Design review of the part built by this model. Coordinates are the model's own, in mm. A direction names the side the tool comes from. Coordinates: 2 decimals unless noted, no trailing zeros. Write each loop counter-clockwise with the first axis right and the second up, starting at its lowest first coordinate (ties: lowest second). Pieces come first, ordered by that corner, then holes. Notation, with made-up numbers: (62, -11) - (109, -11) arc R8 ccw to (109, 3) - close; hole circle Ø10 at (19, 1.5). An arc over 180 degrees is marked (long way). Answer as a JSON object with one key per item and string values.
```python
from build123d import *

# Parameters (mm, degrees)
BOSS_EXTRUDE1_DEPTH      = 25
BOSS_EXTRUDE1_DEPTH_BACK = 25
SKETCH2_W                = 1000
SKETCH2_H                = 25.4
CUT_EXTRUDE1_DEPTH       = 762
CUT_EXTRUDE1_DEPTH_BACK  = 762
SKETCH4_W                = 23.68
SKETCH4_H                = 49.713198884
SKETCH5_R                = 2.45
CUT_EXTRUDE2_DEPTH       = 39.05
CUT_EXTRUDE3_DEPTH       = 39.05
CUT_EXTRUDE3_DEPTH_BACK  = 39.05
SKETCH6_R                = 2.4


with BuildPart() as part:
    # Sketch2 → Boss-Extrude1 (new, two sides: drawn at the far end of the back side and taken through both)
    with BuildSketch(Plane(origin=(0, 0, 0), x_dir=(1, 0, 0), z_dir=(0, 1, 0)).offset(-BOSS_EXTRUDE1_DEPTH_BACK)):
        Rectangle(SKETCH2_W, SKETCH2_H)
    extrude(amount=BOSS_EXTRUDE1_DEPTH + BOSS_EXTRUDE1_DEPTH_BACK)

    # Sketch4 → Cut-Extrude1 (cut, two sides: drawn at the far end of the back side and taken through both)
    with BuildSketch(Plane(origin=(0, 0, 0), x_dir=(0, 0, -1), z_dir=(1, 0, 0)).offset(-CUT_EXTRUDE1_DEPTH_BACK)):
        with Locations((0, -0.716599442)):
            Rectangle(SKETCH4_W, SKETCH4_H)
    extrude(amount=CUT_EXTRUDE1_DEPTH + CUT_EXTRUDE1_DEPTH_BACK, mode=Mode.SUBTRACT)

    # Sketch5 → Cut-Extrude2 (cut)
    with BuildSketch(Plane(origin=(0, 0, 0), x_dir=(1, 0, 0), z_dir=(0, 1, 0))):
        with Locations(Location((0, 0, 0), (0, 0, 90))):
            Circle(SKETCH5_R)
        with Locations(Location((150, 0, 0), (0, 0, 90))):
            Circle(SKETCH5_R)
        with Locations(Location((300, 0, 0), (0, 0, 90))):
            Circle(SKETCH5_R)
        with Locations(Location((450, 0, 0), (0, 0, 90))):
            Circle(SKETCH5_R)
        with Locations(Location((-150, 0, 0), (0, 0, 90))):
            Circle(SKETCH5_R)
        with Locations(Location((-300, 0, 0), (0, 0, 90))):
            Circle(SKETCH5_R)
        with Locations(Location((-450, 0, 0), (0, 0, 90))):
            Circle(SKETCH5_R)
    extrude(amount=CUT_EXTRUDE2_DEPTH, mode=Mode.SUBTRACT)

    # Sketch6 → Cut-Extrude3 (cut, two sides: drawn at the far end of the back side and taken through both)
    with BuildSketch(Plane.XY.offset(-CUT_EXTRUDE3_DEPTH_BACK)):
        with Locations(Location((0, 15, 0), (0, 0, 180))):
            Circle(SKETCH6_R)
        with Locations(Location((0, -15, 0), (0, 0, 180))):
            Circle(SKETCH6_R)
        with Locations(Location((200, 15, 0), (0, 0, 180))):
            Circle(SKETCH6_R)
        with Locations(Location((200, -15, 0), (0, 0, 180))):
            Circle(SKETCH6_R)
        with Locations(Location((400, 15, 0), (0, 0, 180))):
            Circle(SKETCH6_R)
        with Locations(Location((400, -15, 0), (0, 0, 180))):
            Circle(SKETCH6_R)
        with Locations((600, 15)):
            Circle(SKETCH6_R)
        with Locations((600, -15)):
            Circle(SKETCH6_R)
        with Locations(Location((-200, 15, 0), (0, 0, 180))):
            Circle(SKETCH6_R)
        with Locations(Location((-200, -15, 0), (0, 0, 180))):
            Circle(SKETCH6_R)
        with Locations(Location((-400, 15, 0), (0, 0, 180))):
            Circle(SKETCH6_R)
        with Locations(Location((-400, -15, 0), (0, 0, 180))):
            Circle(SKETCH6_R)
        with Locations((-600, 15)):
            Circle(SKETCH6_R)
        with Locations((-600, -15)):
            Circle(SKETCH6_R)
    extrude(amount=CUT_EXTRUDE3_DEPTH + CUT_EXTRUDE3_DEPTH_BACK, mode=Mode.SUBTRACT)


solid = part.part
```
(1) The part is to be moulded in two halves that separate along Z. For faces 1 (the face through (-7, -1, -11.84)), 2 (the face through (-500, 0, -12)), 3 (the face through (-7, 0, -12.7)), 4 (the face through (-7, -1, 11.84)), say which applies: pulls with the +Z half, pulls with the -Z half, needs draft (parallel to the pull), parting line crosses it, or undercut.
Solved:
{"face 1": "undercut", "face 2": "needs draft", "face 3": "pulls with the -Z half", "face 4": "undercut"}
(2) Take a section at B-B, the plane x = 74. Write out the cut boundary in (y, z), and give its area (3 significant figures).
Solved:
{"outline": "(-25, -12.7) - (25, -12.7) - (25, 12.7) - (-25, 12.7) - (-25, 11.84) - (24.14, 11.84) - (24.14, -11.84) - (-25, -11.84) - close", "area": "106 mm^2"}
(3) Take a section at C-C, the plane z = -7.25. Write out the cut boundary in (x, y).
Solved:
{"outline": "(-500, 24.14) - (500, 24.14) - (500, 25) - (-500, 25) - close"}
(4) For pin 1 (8 mm diameter, centred on x = 450, z = 0, fed in from -Y), flat-tipped, find the tip position at first contact; note if it passes through.
Solved:
{"pin 1": "stops at y = 24.14"}
(5) To check wall thickness, follow line 1 (Y direction, x = -400, z = -12.45); line 2 (Z direction, x = -420, y = -9.5); line 3 (Z direction, x = 150, y = 24.45). State the ranges of each line that lie inside material, in increasing order. Write a range as from..to.
Solved:
{"line 1": "y = -25..-17.4, -12.6..12.6, 17.4..25", "line 2": "z = -12.7..-11.84, 11.84..12.7", "line 3": "z = -12.7..-2.45, 2.45..12.7"}
(6) Tool access review of faces 5 (the face through (-7, 24.14, 0)), 6 (the face through (-7, 25, 0)): name each direction out of +Z, -Z, +X, -X, +Y, -Y from which nothing blocks a thin tool from reaching the whole face with its end or side.
Solved:
{"face 5": "+X, -X, -Y", "face 6": "+Z, -Z, +X, -X, +Y"}
(7) Take a section at A-A, the plane y = -2. Write out the cut boundary in (x, z).
Solved:
{"outline": "(-500, -12.7) - (500, -12.7) - (500, -11.84) - (-500, -11.84) - close; (-500, 11.84) - (500, 11.84) - (500, 12.7) - (-500, 12.7) - close"}
